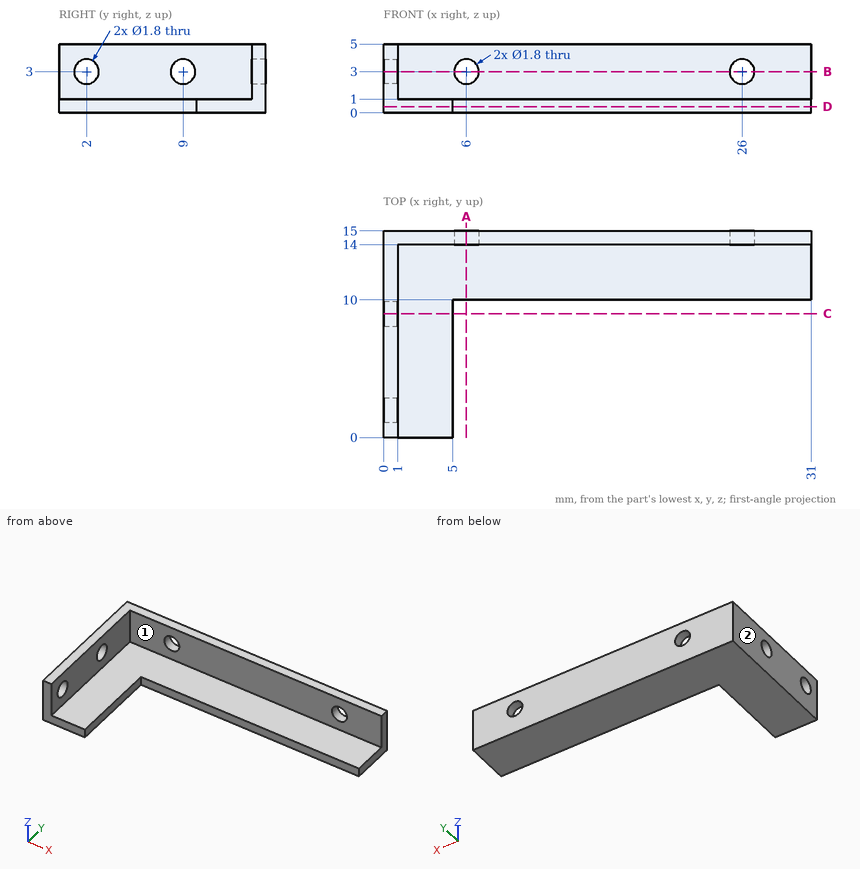
Here's the drawing with two shaded views (mm, measured from the low corner). I have some questions. A direction names the side the tool comes from. Round coordinates to 2 decimals unless told otherwise and drop trailing zeros. Loops run counter-clockwise (first coordinate to the right, second up) from the corner with the lowest first, then second, coordinate; pieces in that order, holes last. Notation, with made-up numbers: (46, 71) - (77, 71) arc R31 ccw to (77, 95) - close; hole circle Ø10 at (-5, -15.5). An arc over 180 degrees is marked (long way). Write item = value, one per line.
1) Imagine slicing it at B-B (z = 3). Please give me the cut outline in (x, y).
Computed:
outline = (0, 0) - (1, 0) - (1, 1.1) - (0, 1.1) - close; (0, 2.9) - (1, 2.9) - (1, 8.1) - (0, 8.1) - close; (0, 9.9) - (1, 9.9) - (1, 14) - (5.1, 14) - (5.1, 15) - (0, 15) - close; (6.9, 14) - (25.1, 14) - (25.1, 15) - (6.9, 15) - close; (26.9, 14) - (31, 14) - (31, 15) - (26.9, 15) - close
2) Imagine slicing it at A-A (x = 6). Please give me the cut outline in (y, z).
Computed:
outline = (10, 0) - (15, 0) - (15, 2.1) - (14, 2.1) - (14, 1) - (10, 1) - close; (14, 3.9) - (15, 3.9) - (15, 5) - (14, 5) - close
3) I need wall thicknesses on line 1 along Y through (x, z) = (0.5, 3); line 2 along X through (y, z) = (5.75, 0.85); line 3 along Y through (x, z) = (11, 2.5). Which ranges of each line are inside material? Lowest first, please. Write a range as from..to.
Computed:
line_1 = 0..1.1, 2.9..8.1, 9.9..15
line_2 = 0..5
line_3 = 14..15
4) On a 3-axis mill with a long thin cutter (end or side, diameter ignored), from which of +Z, -Z, +X, -X, +Y, -Y can I reach the whole of each face in a straight line? I mean the marked faces 1 and 2. Say none if no direction works.
Computed:
face_1 = +Z, +X, -Y
face_2 = +Z, -Z, -X, +Y, -Y
5) Imagine slicing it at C-C (y = 9). Please give me the cut outline in (x, z), and give its area (3 significant figures).
Computed:
outline = (0, 0) - (5, 0) - (5, 1) - (1, 1) - (1, 2.1) - (0, 2.1) - close; (0, 3.9) - (1, 3.9) - (1, 5) - (0, 5) - close
area = 7.20 mm2
6) I'm going to push flat-ended pins straight in: P1, Ø1.5, axis at y = 3.5, z = 4, coming from the +X side; P2, Ø1, axis at x = 12, z = 3, coming from the -Y side; P3, Ø1.4, axis at x = 6, z = 3, coming from the +Y side; P4, Ø0.5, axis at x = 21, z = 0.5, coming from the -Y side. Where does each tip first touch, or does it pass through?
Computed:
P1 = 1
P2 = 14
P3 = through
P4 = 10
7) Imagine slicing it at D-D (z = 0.45). Please give me the cut outline in (x, y), and give its area (3 significant figures).
Computed:
outline = (0, 0) - (5, 0) - (5, 10) - (31, 10) - (31, 15) - (0, 15) - close
area = 205 mm2
